from build123d import *

# Parameters (mm, degrees)
SKETCH1_W               = 25
SKETCH1_H               = 38
BOSS_EXTRUDE1_DEPTH     = 16.5
F_6_32_SLOTS_DEPTH      = 17.5
SKETCH2_11_W            = 5
SKETCH2_11_H            = 5.05
LENS_SEAT_DEPTH         = 3.2
SKETCH2_13_W            = 17.5
SKETCH2_13_H            = 10.1
LENS_PLATE_GROOVE_DEPTH = 8.8
SKETCH6_W               = 25
SKETCH6_H               = 2
ALIGNMENT_GROOVE_DEPTH  = 10
F_4_40_TAPPED_HOLE2_D   = 2.2606


with BuildPart() as part:
    # Sketch1 → Boss-Extrude1 (new body)
    with BuildSketch(Plane(origin=(0, 0, 0), x_dir=(1, 0, 0), z_dir=(0, 1, 0))):
        with Locations((-18481.446731235, 11298.191283293)):
            Rectangle(SKETCH1_W, SKETCH1_H)
    extrude(amount=BOSS_EXTRUDE1_DEPTH)

    # Sketch2 → 6-32 slots (cut, through all)
    with BuildSketch(Plane(origin=(0, 16.5, 0), x_dir=(1, 0, 0), z_dir=(0, 1, 0))):
        with BuildLine():
            Line((-18486.991731235, 11311.691283293), (-18486.991731235, 11308.691283293))
            ThreePointArc((-18486.991731235, 11308.691283293), (-18488.946731235, 11306.736283293), (-18490.901731235, 11308.691283293))
            Line((-18490.901731235, 11308.691283293), (-18490.901731235, 11311.691283293))
            ThreePointArc((-18490.901731235, 11311.691283293), (-18488.946731235, 11313.646283293), (-18486.991731235, 11311.691283293))
        make_face()
        with BuildLine():
            Line((-18486.991731235, 11284.691283293), (-18486.991731235, 11287.691283293))
            ThreePointArc((-18486.991731235, 11287.691283293), (-18488.946731235, 11289.646283293), (-18490.901731235, 11287.691283293))
            Line((-18490.901731235, 11287.691283293), (-18490.901731235, 11284.691283293))
            ThreePointArc((-18490.901731235, 11284.691283293), (-18488.946731235, 11282.736283293), (-18486.991731235, 11284.691283293))
        make_face()
        with BuildLine():
            Line((-18475.901731235, 11284.691283293), (-18475.901731235, 11287.691283293))
            ThreePointArc((-18475.901731235, 11287.691283293), (-18473.946731235, 11289.646283293), (-18471.991731235, 11287.691283293))
            Line((-18471.991731235, 11287.691283293), (-18471.991731235, 11284.691283293))
            ThreePointArc((-18471.991731235, 11284.691283293), (-18473.946731235, 11282.736283293), (-18475.901731235, 11284.691283293))
        make_face()
        with BuildLine():
            Line((-18475.901731235, 11311.691283293), (-18475.901731235, 11308.691283293))
            ThreePointArc((-18475.901731235, 11308.691283293), (-18473.946731235, 11306.736283293), (-18471.991731235, 11308.691283293))
            Line((-18471.991731235, 11308.691283293), (-18471.991731235, 11311.691283293))
            ThreePointArc((-18471.991731235, 11311.691283293), (-18473.946731235, 11313.646283293), (-18475.901731235, 11311.691283293))
        make_face()
    extrude(amount=-F_6_32_SLOTS_DEPTH, mode=Mode.SUBTRACT)

    # Sketch2<11> → lens seat (cut)
    with BuildSketch(Plane(origin=(0, 16.5, 0), x_dir=(1, 0, 0), z_dir=(0, 1, 0))):
        Polygon((-18493.946731235, 11300.191283293), (-18493.946731235, 11298.191283293), (-18488.946731235, 11298.191283293), (-18488.946731235, 11303.241283293), (-18493.946731235, 11303.241283293), align=None)
        with Locations((-18491.446731235, 11295.666283293)):
            Rectangle(SKETCH2_11_W, SKETCH2_11_H)
    extrude(amount=-LENS_SEAT_DEPTH, mode=Mode.SUBTRACT)

    # Sketch2<13> → lens plate groove (cut)
    with BuildSketch(Plane(origin=(0, 16.5, 0), x_dir=(1, 0, 0), z_dir=(0, 1, 0))):
        with Locations((-18477.696731235, 11298.191283293)):
            Rectangle(SKETCH2_13_W, SKETCH2_13_H)
    extrude(amount=-LENS_PLATE_GROOVE_DEPTH, mode=Mode.SUBTRACT)

    # Sketch6 → alignment groove (cut)
    with BuildSketch(Plane(origin=(0, 16.5, 0), x_dir=(1, 0, 0), z_dir=(0, 1, 0))):
        with Locations((-18481.446731235, 11298.191283293)):
            Rectangle(SKETCH6_W, SKETCH6_H)
    extrude(amount=-ALIGNMENT_GROOVE_DEPTH, mode=Mode.SUBTRACT)

    # #4-40 Tapped Hole2 (through all)
    with Locations(Plane(origin=(0, 7.7, 0), x_dir=(1, 0, 0), z_dir=(0, 1, 0))):
        with Locations((-18481.946731235, 11298.191283293)):
            Hole(F_4_40_TAPPED_HOLE2_D / 2)


solid = part.part
Geometry check sheet. Reference: the model listing, model coordinates, mm. A direction names the side the tool comes from. Coordinates: 2 decimals unless noted, no trailing zeros. Order: outer loops, then holes, each group sorted by start corner. A loop starts at its lowest first (then second) coordinate and runs counter-clockwise, first axis right, second up. Notation, with made-up numbers: (66, -0.5) - (99, -0.5) arc R4 cw to (99, 5.5) - close; hole circle Ø7 at (31.25, -29.75). An arc over 180 degrees is marked (long way). Answer in a Markdown table with one row per item. Add a question column.
1) Set-up check for faces 1 (the flat face through (-18490.902, 8, -11310)), 2 (the flat face through (-18488, 6.5, -11298)), 3 (the flat face through (-18478, 12, -11293.141)), 4 (the flat face through (-18491, 15, -11303.241)), 5 (the flat face through (-18468.947, 6, -11298)): record each of +Z, -Z, +X, -X, +Y, -Y from which the full face is reachable in a straight line by a thin tool's end or side.
2) Release check for a two-part mould opening along Z. For faces 6 (the flat face through (-18479, 0, -11298)), 7 (the flat face through (-18482, 8, -11317.191)), 8 (the cylindrical face through (-18481.7, 3.8, -11297.09)) record: +Z half, -Z half, draft (parallel to the pull), parting line (faces both ways), or undercut.
3) Material ranges on line 1 along X through (y, z) = (12, -11286.5); line 2 along Z through (x, y) = (-18484, 11.5); line 3 along X through (y, z) = (15.5, -11283), recorded low to high. Write a range as [from, to].
4) Gauge pin test, flat ends, axial feed: P1, Ø2, axis at x = -18491.5, z = -11295, coming from the +Y side; P2, Ø1.2, axis at x = -18473.5, z = -11296, coming from the +Y side; P3, Ø1, axis at x = -18476.5, z = -11298.5, coming from the +Y side; P4, Ø2, axis at x = -18481.95, z = -11298.19, coming from the +Y side. Record the tip position at first contact, or that the pin passes through.
5) Cross-section at D-D, the plane y = 14.5. State how many separate pieces and enclosed holes the cut face has, then the cut area to 3 significant figures.
6) Cross-section at A-A, the plane y = 12.75. Record the cut outline in (x, z) (3 decimals).
7) Cross-section at B-B, the plane z = -11311. Record the cut outline in (x, y), then the cut area to 3 significant figures.
8) Cross-section at C-C, the plane x = -18478.25. Record the cut outline in (y, z), then the cut area to 3 significant figures.
Check result:
| question | item | result |
|---|---|---|
| 1 | face 1 | +Y, -Y |
| 1 | face 2 | +X, -X, +Y |
| 1 | face 3 | +X, +Y |
| 1 | face 4 | -X, +Y |
| 1 | face 5 | +Z, -Z, +X, +Y, -Y |
| 2 | face 6 | draft |
| 2 | face 7 | -Z half |
| 2 | face 8 | undercut |
| 3 | line 1 | x = [-18493.95, -18490.9], [-18486.99, -18475.9], [-18471.99, -18468.95] |
| 3 | line 2 | z = [-11317.19, -11303.24], [-11293.14, -11279.19] |
| 3 | line 3 | x = [-18493.95, -18489.93], [-18487.97, -18474.93], [-18472.97, -18468.95] |
| 4 | P1 | stops at y = 13.3 |
| 4 | P2 | stops at y = 7.7 |
| 4 | P3 | stops at y = 6.5 |
| 4 | P4 | passes through |
| 5 | separate pieces | 2 |
| 5 | enclosed holes | 4 |
| 5 | area | 623 mm² |
| 6 | outline | (-18493.947, -11317.191) - (-18468.947, -11317.191) - (-18468.947, -11303.241) - (-18486.447, -11303.241) - (-18486.447, -11299.191) - (-18493.947, -11299.191) - close; (-18493.947, -11297.191) - (-18486.447, -11297.191) - (-18486.447, -11293.141) - (-18468.947, -11293.141) - (-18468.947, -11279.191) - (-18493.947, -11279.191) - close; hole (-18490.902, -11311.691) arc R1.955 ccw to (-18486.992, -11311.691) - (-18486.992, -11308.691) arc R1.955 ccw to (-18490.902, -11308.691) - close; hole (-18490.902, -11287.691) arc R1.955 ccw to (-18486.992, -11287.691) - (-18486.992, -11284.691) arc R1.955 ccw to (-18490.902, -11284.691) - close; hole (-18475.902, -11311.691) arc R1.955 ccw to (-18471.992, -11311.691) - (-18471.992, -11308.691) arc R1.955 ccw to (-18475.902, -11308.691) - close; hole (-18475.902, -11287.691) arc R1.955 ccw to (-18471.992, -11287.691) - (-18471.992, -11284.691) arc R1.955 ccw to (-18475.902, -11284.691) - close |
| 7 | outline | (-18493.95, 0) - (-18490.9, 0) - (-18490.9, 16.5) - (-18493.95, 16.5) - close; (-18486.99, 0) - (-18475.9, 0) - (-18475.9, 16.5) - (-18486.99, 16.5) - close; (-18471.99, 0) - (-18468.95, 0) - (-18468.95, 16.5) - (-18471.99, 16.5) - close |
| 7 | area | 283 mm² |
| 8 | outline | (0, -11317.19) - (16.5, -11317.19) - (16.5, -11303.24) - (7.7, -11303.24) - (7.7, -11299.19) - (6.5, -11299.19) - (6.5, -11297.19) - (7.7, -11297.19) - (7.7, -11293.14) - (16.5, -11293.14) - (16.5, -11279.19) - (0, -11279.19) - close |
| 8 | area | 536 mm² |
